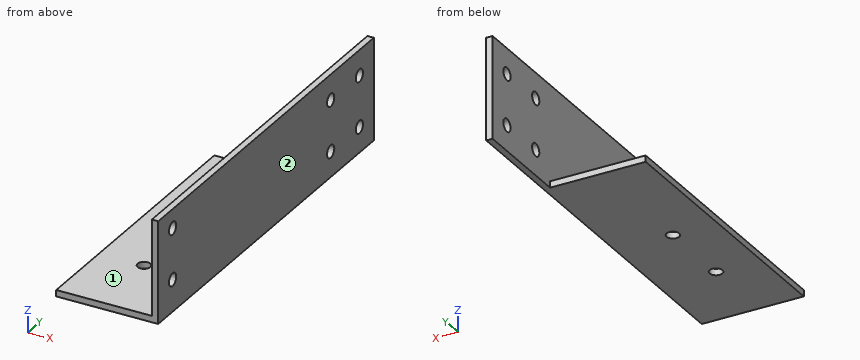
Autodesk Inventor part; units mm, degrees
ref_plane "YZ Plane" through (0, 0, 0) normal (1, 0, 0) x (0, 1, 0)
ref_plane "XZ Plane" through (0, 0, 0) normal (0, 1, 0) x (-1, 0, 0)
ref_plane "XY Plane" through (0, 0, 0) normal (0, 0, 1) x (1, 0, 0)
sketch "Sketch1" plane through (0, 0, 0) normal (0, 1, 0) x (-1, 0, 0)
  line L0 (0, 0) -> (3.175, 0)
  line L1 (3.175, 0) -> (3.175, 50.8)
  line L2 (3.175, 50.8) -> (0, 50.8)
  line L3 (0, 50.8) -> (0, 0)
  line L4 (0, 0) -> (50.8, 0)
  line L5 (50.8, 0) -> (50.8, 3.175)
  line L6 (50.8, 3.175) -> (0, 3.175)
  line L7 (0, 3.175) -> (0, 0)
  dimension "d0" = 3.175
  dimension "d1" = 50.8
  dimension "d2" = 50.8
  dimension "d3" = 3.175
extrude "Extrusion1" add sketch "Sketch1" against normal blind 139.7
sketch "Sketch3" plane through (0, 0, 50.8) normal (1, 0, 0) x (0, 0, -1)
  line L0 (50.8, -139.7) -> (0, -139.7)
  line L1 (50.8, 0) -> (50.8, -139.7)
  line L2 (0, 0) -> (50.8, 0)
  line L3 (0, 0) -> (0, -139.7)
  point P0 (9.525, -127)
  point P1 (34.925, -127)
  dimension "d17" = 12.7
  dimension "d18" = 9.525
  dimension "d19" = 15.875
  dimension "d20" = 12.7
hole "Hole2" at (0, -127, 41.275) at (0, -127, 15.875) direction (-1, 0, 0) diameter 6.35 end through all
sketch "Sketch4" plane through (0, 0, 0) normal (0, 0, -1) x (-1, 0, 0)
  line L0 (0, 0) -> (50.8, 0)
  line L1 (0, 0) -> (0, -139.7)
  line L2 (50.8, -139.7) -> (0, -139.7)
  line L3 (50.8, 0) -> (50.8, -139.7)
  point P0 (28.575, -63.5)
  point P1 (28.575, -101.6)
  dimension "d28" = 28.575
  dimension "d29" = 63.5
  dimension "d30" = 101.6
  dimension "d31" = 28.575
hole "Hole3" at (-28.575, -63.5, 0) at (-28.575, -101.6, 0) direction (0, 0, 1) diameter 6.35 end through all
sketch "Sketch5" plane through (0, 0, 0) normal (0, 1, 0) x (1, 0, 0)
  line L0 (0, 0) -> (-3.175, 0)
  line L1 (-3.175, 0) -> (-3.175, -50.8)
  line L2 (-3.175, -50.8) -> (0, -50.8)
  line L3 (0, -50.8) -> (0, 0)
extrude "Extrusion2" add sketch "Sketch5" along normal blind 50.8
sketch "Sketch6" plane through (0, -139.7, 50.8) normal (1, 0, 0) x (0, 0, -1)
  circle A0 centre (9.525, 12.7) radius 3.175
  circle A1 centre (34.925, 12.7) radius 3.175
  line L0 (0, 0) -> (0, 190.5)
  line L1 (50.8, 0) -> (0, 0)
  line L2 (50.8, 190.5) -> (50.8, 0)
  line L3 (0, 190.5) -> (50.8, 190.5)
  point P0 (50.8, 139.7)
  point P1 (12.7, 152.4)
  point P2 (38.1, 152.4)
  point P3 (12.7, 177.8)
  point P4 (38.1, 177.8)
  dimension "d41" = 38.1
  dimension "d42" = 12.7
  dimension "d43" = 12.7
  dimension "d44" = 38.1
  dimension "d45" = 12.7
  dimension "d46" = 12.7
  dimension "d47" = 12.7
  dimension "d48" = 12.7
hole "Hole4" at (0, 12.7, 38.1) at (0, 12.7, 12.7) at (0, 38.1, 38.1) at (0, 38.1, 12.7) direction (-1, 0, 0) diameter 6.35 end through all
properties part number "2x2 angle vertical right"
Design review of the part built by this model. Coordinates are the model's own, in mm. Face numbers are marked on the shaded views. A direction names the side the tool comes from. Give positions to 0.01 mm unless a question says otherwise; leave off trailing zeros. Write each loop counter-clockwise with the first axis right and the second up, starting at its lowest first coordinate (ties: lowest second). Pieces come first, ordered by that corner, then holes. Notation, with made-up numbers: M 72,-36 L 84,-36 A19 ccw 84,-7 Z; hole C 24.5,-17.75 d11. An arc over 180 degrees is marked long. Answer as a JSON object with one key per item and string values. Group by question number.
1) We need section D-D (z = 5). Give the boundary of the cut face in (x, y) (3 decimals).
2) Clearance check with flat-ended pins moving along their axes: pin 1 Ø24 at (x, y) = (-21.5, -56.5) entering from +Z (3 decimals); pin 2 Ø10 at (y, z) = (-127, 41.275) entering from -X (3 decimals); pin 3 Ø2.5 at (x, z) = (-37, 1) entering from +Y. State where each tip first meets the part, or that it passes through.
3) For line 1 along Z through (x, y) = (-2.1, 38.1) (3 decimals); line 2 along Z through (x, y) = (-2, -127); line 3 along X through (y, z) = (-101.6, 2.3), list the stretches that pass through material, from the lowest coordinate up.
4) Tool access review of the marked faces 1 and 2: name each direction out of +Z, -Z, +X, -X, +Y, -Y from which nothing blocks a thin tool from reaching the whole face with its end or side.
5) We need section C-C (y = 12.7). Give the boundary of the cut face in (x, z) (3 decimals), and give its area (3 significant figures).
6) We need section B-B (y = -63.5). Give the boundary of the cut face in (x, z) (3 decimals).
7) We need section A-A (y = -127). Give the boundary of the cut face in (x, z) (3 decimals), and give its area (3 significant figures).
Answer key:
{
 "1": {"outline": "M -3.175,-139.7 L 0,-139.7 L 0,50.8 L -3.175,50.8 Z"},
 "2": {"pin 1": "stops at z = 3.175", "pin 2": "stops at x = -3.175", "pin 3": "stops at y = 0"},
 "3": {"line 1": "z = 0 to 9.525, 15.875 to 34.925, 41.275 to 50.8", "line 2": "z = 0 to 12.7, 19.05 to 38.1, 44.45 to 50.8", "line 3": "x = -50.8 to -31.75, -25.4 to 0"},
 "4": {"face 1": "+Z, -X, +Y, -Y", "face 2": "+Z, -Z, +X, +Y, -Y"},
 "5": {"outline": "M -3.175,0 L 0,0 L 0,9.525 L -3.175,9.525 Z; M -3.175,15.875 L 0,15.875 L 0,34.925 L -3.175,34.925 Z; M -3.175,41.275 L 0,41.275 L 0,50.8 L -3.175,50.8 Z", "area": "121 mm²"},
 "6": {"outline": "M -50.8,0 L -31.75,0 L -31.75,3.175 L -50.8,3.175 Z; M -25.4,0 L 0,0 L 0,50.8 L -3.175,50.8 L -3.175,3.175 L -25.4,3.175 Z"},
 "7": {"outline": "M -50.8,0 L 0,0 L 0,12.7 L -3.175,12.7 L -3.175,3.175 L -50.8,3.175 Z; M -3.175,19.05 L 0,19.05 L 0,38.1 L -3.175,38.1 Z; M -3.175,44.45 L 0,44.45 L 0,50.8 L -3.175,50.8 Z", "area": "272 mm²"}
}
